Here's how the part is built. I have some questions about the finished solid (model axes, mm). Round coordinates to 2 decimals unless told otherwise and drop trailing zeros. Order: outer loops, then holes, each group sorted by start corner. A loop starts at its lowest first (then second) coordinate and runs counter-clockwise, first axis right, second up. Notation, with made-up numbers: (2, 75.5) -> (19, 75.5) arc R26 ccw to (19, 97.5) -> close; hole circle Ø10 at (73.5, 13.5). An arc over 180 degrees is marked (long way). Answer in a Markdown table with one row per item.
```python
from build123d import *

# Parameters (mm, degrees)
F0_W     = 48.50465
F0_H     = 123.528182
F0_R     = 14.869819
F1_DEPTH = 6.35
F2_R     = 8.89
F3_DEPTH = 6.351


with BuildPart() as f1:
    # F0 (on Top) → F1 (new body)
    with BuildSketch(Plane.XY):
        Rectangle(F0_W, F0_H)
        with Locations((0, -41.818257)):
            Circle(F0_R, mode=Mode.SUBTRACT)
    extrude(amount=F1_DEPTH)

    # F2 (on face) → F3 (cut, through all)
    with BuildSketch(Plane.XY.offset(6.35)):
        with Locations((17.947458, 45.703962)):
            Circle(F2_R)
        with Locations((18.347179, 20.307108)):
            Circle(F2_R)
        with Locations((18.7469, -5.089747)):
            Circle(F2_R)
    extrude(amount=-F3_DEPTH, mode=Mode.SUBTRACT)


solid = f1.part
```
1. Suppose I cut it at B-B on z = 2.25. Write out the boundary of the cut face in (x, y).
Numbers:
| item | result |
|---|---|
| outline | (-24.25, -61.76) -> (24.25, -61.76) -> (24.25, -12.07) arc R8.89 cw (long way) to (24.25, 1.89) -> (24.25, 13.66) arc R8.89 cw (long way) to (24.25, 26.95) -> (24.25, 39.44) arc R8.89 cw (long way) to (24.25, 51.97) -> (24.25, 61.76) -> (-24.25, 61.76) -> close; hole circle Ø29.74 at (0, -41.82) |
2. Please list where these lines run through material, in increasing order: line 1 along Y through (x, z) = (11, 1.25); line 2 along Y through (x, z) = (0, 5); line 3 along Y through (x, z) = (7.5, 5.75).
Numbers:
| item | result |
|---|---|
| line 1 | y = -61.76 to -51.82, -31.81 to -9.45, -0.73 to 15.3, 25.31 to 40.16, 51.25 to 61.76 |
| line 2 | y = -61.76 to -56.69, -26.95 to 61.76 |
| line 3 | y = -61.76 to -54.66, -28.98 to 61.76 |
3. Suppose I cut it at A-A on x = 0. Write out the boundary of the cut face in (y, z), then the cut area to 3 significant figures.
Numbers:
| item | result |
|---|---|
| outline | (-61.76, 0) -> (-56.69, 0) -> (-56.69, 6.35) -> (-61.76, 6.35) -> close; (-26.95, 0) -> (61.76, 0) -> (61.76, 6.35) -> (-26.95, 6.35) -> close |
| area | 596 mm2 |
4. Suppose I cut it at C-C on x = -7. Write out the boundary of the cut face in (y, z).
Numbers:
| item | result |
|---|---|
| outline | (-61.76, 0) -> (-54.94, 0) -> (-54.94, 6.35) -> (-61.76, 6.35) -> close; (-28.7, 0) -> (61.76, 0) -> (61.76, 6.35) -> (-28.7, 6.35) -> close |
5. Suppose I cut it at D-D on y = 0. Write out the boundary of the cut face in (x, z).
Numbers:
| item | result |
|---|---|
| outline | (-24.25, 0) -> (11.46, 0) -> (11.46, 6.35) -> (-24.25, 6.35) -> close |
